Drawing for the job (mm, zero at the part's lowest x, y, z). A direction names the side the tool comes from. Round coordinates to 2 decimals unless told otherwise and drop trailing zeros. Loops run counter-clockwise (first coordinate to the right, second up) from the corner with the lowest first, then second, coordinate; pieces in that order, holes last. Notation, with made-up numbers: M 26.25,19.5 L 32.25,19.5 A24 cw 32.25,51.5 Z; hole C 56.25,-33 d1. An arc over 180 degrees is marked long. Put each result on its own line as item: value. Start each with the question number.
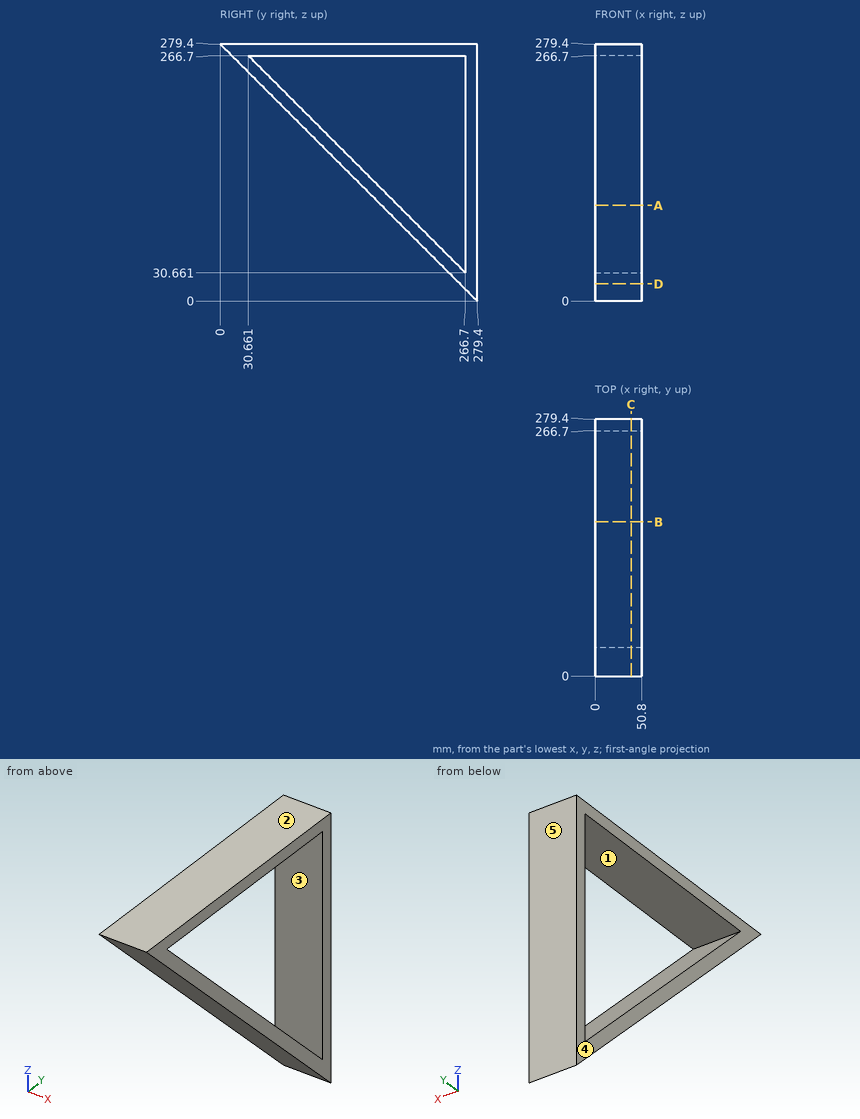
1. Cut at A-A, the plane z = 104. Give the cut face in (x, y).
2. Wall check: L1, parallel to Z at x = 48, y = 228; L2, parallel to Y at x = 28.5, z = 179; L3, parallel to Z at x = 33, y = 203. Give the ranges that are in metal, low to high.
3. Cut at C-C, the plane x = 39. Give the cut face in (y, z), and give its area (3 significant figures).
4. Drop flat-ended pins along their axis: pin 1 (15 mm diameter, centred on x = 27, z = 197.5, fed in from -Y); pin 2 (2 mm diameter, centred on x = 18, y = 136, fed in from -Z); pin 3 (1.5 mm diameter, centred on x = 13, z = 61.5, fed in from -Y). Give the stop position or say it passes through.
5. Mould opens along Y. For the marked faces 3, 4 and 5 say: released by +Y, released by -Y, zero draft, split by the parting line, or undercut.
6. Cut at D-D, the plane z = 18.5. Give the cut face in (x, y), and give its area (3 significant figures).
7. Which spindle directions (+Z, -Z, +X, -X, +Y, -Y) get a long thin tool onto all of the face, cutting with end or side? Do the marked faces 1 and 2. Say none if no direction does.
8. Cut at B-B, the plane y = 167.5. Give the cut face in (x, z).
Results list:
1. outline: M 0,175.4 L 50.8,175.4 L 50.8,193.36 L 0,193.36 Z; M 0,266.7 L 50.8,266.7 L 50.8,279.4 L 0,279.4 Z
2. L1: z = 51.4 to 69.36, 266.7 to 279.4
2. L2: y = 100.4 to 118.36, 266.7 to 279.4
2. L3: z = 76.4 to 94.36, 266.7 to 279.4
3. outline: M 0,279.4 L 279.4,0 L 279.4,279.4 Z; hole M 30.66,266.7 L 266.7,30.66 L 266.7,266.7 Z
3. area: 11,200 mm^2
4. pin 1: stops at y = 74.4
4. pin 2: stops at z = 142.4
4. pin 3: stops at y = 217.15
5. face 3: undercut
5. face 4: zero draft
5. face 5: released by +Y
6. outline: M 0,260.9 L 50.8,260.9 L 50.8,279.4 L 0,279.4 Z
6. area: 940 mm^2
7. face 1: +X, -X
7. face 2: +Z, +X, -X, +Y, -Y
8. outline: M 0,111.9 L 50.8,111.9 L 50.8,129.86 L 0,129.86 Z; M 0,266.7 L 50.8,266.7 L 50.8,279.4 L 0,279.4 Z
